Check sheet for the modelled part. Datum: model origin and axes. Units: mm. Face numbers are marked on the shaded views. A direction names the side the tool comes from. Round coordinates to 2 decimals unless told otherwise and drop trailing zeros. Loops run counter-clockwise (first coordinate to the right, second up) from the corner with the lowest first, then second, coordinate; pieces in that order, holes last. Notation, with made-up numbers: (36.25, -5.75) - (73.25, -5.75) arc R18 cw to (73.25, 29.25) - close; hole circle Ø8 at (-3.75, 16). An arc over 180 degrees is marked (long way). Put each result on its own line as item: value. Start each with the question number.
Item 1: Material ranges on line 1 along Y through (x, z) = (61.5, 49.4); line 2 along X through (y, z) = (407.5, 48.55); line 3 along X through (y, z) = (474.5, 46.75), recorded low to high.
Item 2: Section check C-C, the plane x = 82.5. Record the cut outline in (y, z), and give its area (3 significant figures).
Item 3: Section check A-A, the plane z = 48.75. Give the number of separate pieces and of enclosed holes in the cut face, and give its area (3 significant figures).
Item 4: Tool access check on the marked faces 1, 2 and 3. Record the directions out of +Z, -Z, +X, -X, +Y, -Y that give a thin tool (end or side, any length) a straight path to the whole face; none if there is none.
Item 5: Gauge pin test, flat end, axial feed: pin 1 Ø1 at (x, y) = (58, 455) entering from -Z. Record the tip position at first contact, or that the pin passes through.
Item 6: Section check B-B, the plane y = 378. Record the cut outline in (x, z), and give its area (3 significant figures).
from build123d import *

# Parameters (mm, degrees)
BOX033_W          = 5
BOX033_H          = 22
BOX033_DEPTH      = 5
ARRAY004_Y_COUNT  = 5
ARRAY004_Y_PITCH  = 35
BOX032_W          = 5
BOX032_H          = 22
BOX032_DEPTH      = 5
ARRAY003_Y_COUNT  = 5
ARRAY003_Y_PITCH  = 35
CYLINDER012_R     = 2
CYLINDER012_DEPTH = 196
BOX031_W          = 50
BOX031_H          = 196
BOX031_DEPTH      = 3


with BuildPart() as array004:
    # Box033 → Box033 (new body)
    with BuildSketch(Plane.XY):
        with Locations((2.5, 11)):
            Rectangle(BOX033_W, BOX033_H)
    extrude(amount=BOX033_DEPTH)

    # Array004 Y: Array004 ×5


with BuildPart() as array004_1:
    add(array004.part)
    with Locations(*[(0, i * ARRAY004_Y_PITCH, 0) for i in range(1, ARRAY004_Y_COUNT)]):
        add(array004.part)


with BuildPart() as array004_2:
    # Array004 placement: moved
    add(array004_1.part.moved(Location((88, 318, 47))))


with BuildPart() as array003:
    # Box032 → Box032 (new body)
    with BuildSketch(Plane.XY):
        with Locations((2.5, 11)):
            Rectangle(BOX032_W, BOX032_H)
    extrude(amount=BOX032_DEPTH)

    # Array003 Y: Array003 ×5


with BuildPart() as array003_1:
    add(array003.part)
    with Locations(*[(0, i * ARRAY003_Y_PITCH, 0) for i in range(1, ARRAY003_Y_COUNT)]):
        add(array003.part)


with BuildPart() as array003_2:
    # Array003 placement: moved
    add(array003_1.part.moved(Location((57, 318, 47))))


with BuildPart() as obj1:
    # Cylinder012 → Cylinder012 (new body)
    with BuildSketch(Plane(origin=(75, 498, 47), x_dir=(1, 0, 0), z_dir=(0, -1, 0))):
        Circle(CYLINDER012_R)
    extrude(amount=CYLINDER012_DEPTH)


with BuildPart() as soporte_electronica_con_agujeros:
    # Box031 → Box031 (new body)
    with BuildSketch(Plane(origin=(50, 302, 47), x_dir=(1, 0, 0), z_dir=(0, 0, 1))):
        with Locations((25, 98)):
            Rectangle(BOX031_W, BOX031_H)
    extrude(amount=BOX031_DEPTH)

    # Fusion012: union obj1
    add(obj1.part)

    # Cut021005: cut Array003
    add(array003_2.part, mode=Mode.SUBTRACT)

    # Cut021006: cut Array004
    add(array004_2.part, mode=Mode.SUBTRACT)


solid = soporte_electronica_con_agujeros.part
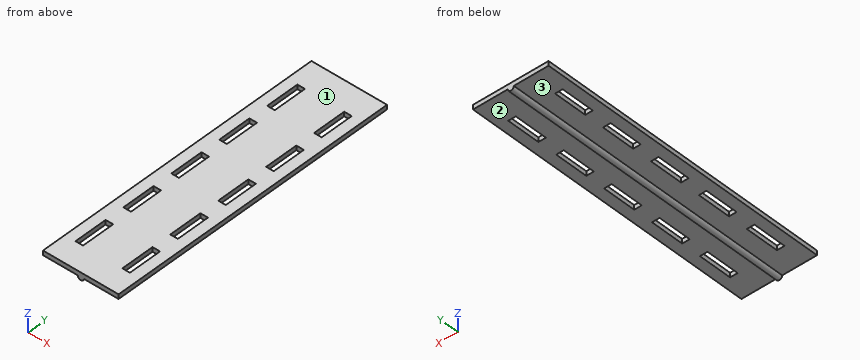
Check result:
1. line 1: 302 to 318, 340 to 353, 375 to 388, 410 to 423, 445 to 458, 480 to 498
1. line 2: 50 to 57, 62 to 88, 93 to 100
1. line 3: 73.02 to 76.98
2. outline: (302, 47) - (498, 47) - (498, 50) - (302, 50) - close
2. area: 588 mm²
3. separate pieces: 1
3. enclosed holes: 10
3. area: 8,700 mm²
4. face 1: +Z, +X, -X, +Y, -Y
4. face 2: -Z, +X, +Y, -Y
4. face 3: -Z, -X, +Y, -Y
5. pin 1: z = 47
6. outline: (50, 47) - (73, 47) arc R2 ccw to (77, 47) - (100, 47) - (100, 50) - (50, 50) - close
6. area: 156 mm²
